Geometry check sheet. Reference: the model listing, model coordinates, mm. A direction names the side the tool comes from. Coordinates: 2 decimals unless noted, no trailing zeros. Loops run counter-clockwise (first coordinate to the right, second up) from the corner with the lowest first, then second, coordinate; pieces in that order, holes last. Notation, with made-up numbers: (28, 45) - (72, 45) arc R4 cw to (72, 50) - close; hole circle Ø6 at (24.25, 26). An arc over 180 degrees is marked (long way). Write item = value, one per line. Start each with the question number.
from build123d import *

# Parameters (mm, degrees)
SKETCH1_W                     = 114.3
SKETCH1_H                     = 254
BOSS_EXTRUDE1_DEPTH           = 2.000000064
M4_CLEARANCE_HOLE1_AT_2_COUNT = 2
M4_CLEARANCE_HOLE1_AT_2_PITCH = 64.13133097
M4_CLEARANCE_HOLE1_AT_3_COUNT = 2
M4_CLEARANCE_HOLE1_AT_3_PITCH = 171.44126128
M4_CLEARANCE_HOLE1_AT_4_COUNT = 2
M4_CLEARANCE_HOLE1_AT_4_PITCH = 158.994586252
SKETCH8_R                     = 6.35
BOSS_EXTRUDE3_DEPTH           = 3


with BuildPart() as part:
    # Sketch1 → Boss-Extrude1 (new body)
    with BuildSketch(Plane(origin=(0, 0, 0), x_dir=(1, 0, 0), z_dir=(0, 1, 0))):
        with Locations((57.15, 127)):
            Rectangle(SKETCH1_W, SKETCH1_H)
    extrude(amount=BOSS_EXTRUDE1_DEPTH)

    # Sketch6 → M4 Clearance Hole1 (revolve, cut)
    with BuildSketch(Plane(origin=(25.146, 2.000000064, -206.502), x_dir=(0, 0, 1), z_dir=(1, 0, 0))):
        Polygon((0, 0), (0, 2.000000064), (2.25, 2.000000064), (2.25, 0.025), (2.275, 0), align=None)
    m4_clearance_hole1 = revolve(axis=Axis((25.146, 8.350000064, -206.502), (0, -1, 0)), mode=Mode.SUBTRACT)

    # M4 Clearance Hole1 at 2: M4 Clearance Hole1 ×2
    with Locations(*[(i * M4_CLEARANCE_HOLE1_AT_2_PITCH, 0, 0) for i in range(1, M4_CLEARANCE_HOLE1_AT_2_COUNT)]):
        add(m4_clearance_hole1, mode=Mode.SUBTRACT)

    # M4 Clearance Hole1 at 3: M4 Clearance Hole1 ×2
    with Locations(*[Vector(0.37407174, 0, 0.92739977) * (i * M4_CLEARANCE_HOLE1_AT_3_PITCH) for i in range(1, M4_CLEARANCE_HOLE1_AT_3_COUNT)]):
        add(m4_clearance_hole1, mode=Mode.SUBTRACT)

    # M4 Clearance Hole1 at 4: M4 Clearance Hole1 ×2
    with Locations(*[(0, 0, i * M4_CLEARANCE_HOLE1_AT_4_PITCH) for i in range(1, M4_CLEARANCE_HOLE1_AT_4_COUNT)]):
        add(m4_clearance_hole1, mode=Mode.SUBTRACT)

    # Sketch8 → Boss-Extrude3 (add)
    with BuildSketch(Plane(origin=(0, 2.000000064, 0), x_dir=(1, 0, 0), z_dir=(0, 1, 0))):
        with Locations((89.27733097, 47.507413748)):
            Circle(SKETCH8_R)
        with BuildLine():
            ThreePointArc((89.228972354, 43.291716477), (89.012687116, 43.241374316), (88.800207525, 43.305919345))
            Line((88.800207525, 43.305919345), (85.540585246, 45.334637149))
            ThreePointArc((85.540585246, 45.334637149), (85.388845037, 45.496774579), (85.338502876, 45.713059817))
            Line((85.338502876, 45.713059817), (85.465612892, 49.55033442))
            ThreePointArc((85.465612892, 49.55033442), (85.53015792, 49.762814011), (85.692295351, 49.91455422))
            Line((85.692295351, 49.91455422), (89.079027646, 51.723111019))
            ThreePointArc((89.079027646, 51.723111019), (89.295312884, 51.77345318), (89.507792475, 51.708908151))
            Line((89.507792475, 51.708908151), (92.767414754, 49.680190347))
            ThreePointArc((92.767414754, 49.680190347), (92.919154963, 49.518052917), (92.969497124, 49.301767679))
            Line((92.969497124, 49.301767679), (92.842387108, 45.464493076))
            ThreePointArc((92.842387108, 45.464493076), (92.77784208, 45.252013485), (92.615704649, 45.100273276))
            Line((92.615704649, 45.100273276), (89.228972354, 43.291716477))
        make_face(mode=Mode.SUBTRACT)
        with Locations((25.02266903, 47.507413748)):
            Circle(SKETCH8_R)
        with BuildLine():
            Line((28.759414754, 45.334637149), (25.499792475, 43.305919345))
            ThreePointArc((25.499792475, 43.305919345), (25.287312884, 43.241374316), (25.071027646, 43.291716477))
            Line((25.071027646, 43.291716477), (21.684295351, 45.100273276))
            ThreePointArc((21.684295351, 45.100273276), (21.52215792, 45.252013485), (21.457612892, 45.464493076))
            Line((21.457612892, 45.464493076), (21.330502876, 49.301767679))
            ThreePointArc((21.330502876, 49.301767679), (21.380845037, 49.518052917), (21.532585246, 49.680190347))
            Line((21.532585246, 49.680190347), (24.792207525, 51.708908151))
            ThreePointArc((24.792207525, 51.708908151), (25.004687116, 51.77345318), (25.220972354, 51.723111019))
            Line((25.220972354, 51.723111019), (28.607704649, 49.91455422))
            ThreePointArc((28.607704649, 49.91455422), (28.76984208, 49.762814011), (28.834387108, 49.55033442))
            Line((28.834387108, 49.55033442), (28.961497124, 45.713059817))
            ThreePointArc((28.961497124, 45.713059817), (28.911154963, 45.496774579), (28.759414754, 45.334637149))
        make_face(mode=Mode.SUBTRACT)
        with Locations((89.27733097, 206.492586252)):
            Circle(SKETCH8_R)
        with BuildLine():
            Line((89.228972354, 210.708283523), (92.615704649, 208.899726724))
            ThreePointArc((92.615704649, 208.899726724), (92.77784208, 208.747986515), (92.842387108, 208.535506924))
            Line((92.842387108, 208.535506924), (92.969497124, 204.698232321))
            ThreePointArc((92.969497124, 204.698232321), (92.919154963, 204.481947083), (92.767414754, 204.319809653))
            Line((92.767414754, 204.319809653), (89.507792475, 202.291091849))
            ThreePointArc((89.507792475, 202.291091849), (89.295312884, 202.22654682), (89.079027646, 202.276888981))
            Line((89.079027646, 202.276888981), (85.692295351, 204.08544578))
            ThreePointArc((85.692295351, 204.08544578), (85.53015792, 204.237185989), (85.465612892, 204.44966558))
            Line((85.465612892, 204.44966558), (85.338502876, 208.286940183))
            ThreePointArc((85.338502876, 208.286940183), (85.388845037, 208.503225421), (85.540585246, 208.665362851))
            Line((85.540585246, 208.665362851), (88.800207525, 210.694080655))
            ThreePointArc((88.800207525, 210.694080655), (89.012687116, 210.758625684), (89.228972354, 210.708283523))
        make_face(mode=Mode.SUBTRACT)
        with Locations((25.02266903, 206.492586252)):
            Circle(SKETCH8_R)
        with BuildLine():
            ThreePointArc((25.071027646, 210.708283523), (25.287312884, 210.758625684), (25.499792475, 210.694080655))
            Line((25.499792475, 210.694080655), (28.759414754, 208.665362851))
            ThreePointArc((28.759414754, 208.665362851), (28.911154963, 208.503225421), (28.961497124, 208.286940183))
            Line((28.961497124, 208.286940183), (28.834387108, 204.44966558))
            ThreePointArc((28.834387108, 204.44966558), (28.76984208, 204.237185989), (28.607704649, 204.08544578))
            Line((28.607704649, 204.08544578), (25.220972354, 202.276888981))
            ThreePointArc((25.220972354, 202.276888981), (25.004687116, 202.22654682), (24.792207525, 202.291091849))
            Line((24.792207525, 202.291091849), (21.532585246, 204.319809653))
            ThreePointArc((21.532585246, 204.319809653), (21.380845037, 204.481947083), (21.330502876, 204.698232321))
            Line((21.330502876, 204.698232321), (21.457612892, 208.535506924))
            ThreePointArc((21.457612892, 208.535506924), (21.52215792, 208.747986515), (21.684295351, 208.899726724))
            Line((21.684295351, 208.899726724), (25.071027646, 210.708283523))
        make_face(mode=Mode.SUBTRACT)
    extrude(amount=BOSS_EXTRUDE3_DEPTH)


solid = part.part
(1) Sectioned sample at C-C on x = 64.5. Enter the section's corners in (y, z), plus the area to 3 significant figures.
(2) Scan lines: line 1 (Z direction, x = 89, y = 3.9); line 2 (Z direction, x = 92.5, y = 3.7); line 3 (Y direction, x = 79.5, z = -96). Record each from-to range of solid material in increasing order.
(3) Sectioned sample at B-B on y = 3.5. Count the separate pieces of the cut face and the enclosed holes in it, plus the area to 3 significant figures.
(4) Tool access check on faces 1 (the face through (27.34, 1, -48)), 2 (the face through (26.8, 2, -45.7)). Record the directions out of +Z, -Z, +X, -X, +Y, -Y that give a thin tool (end or side, any length) a straight path to the whole face; none if there is none.
(5) Sectioned sample at A-A on z = -226.5. Enter the section's corners in (x, y).
(6) Draft check along Z on faces 3 (the face through (18.68, 3.48, -47.79)), 4 (the face through (92, 5, -209.4)). Enter one of: pulls with the +Z half, pulls with the -Z half, needs draft (parallel to the pull), parting line crosses it, or undercut.
(7) Depth check by flat-ended pin: pin 1 (4 mm diameter, centred on x = 26.5, z = -206, fed in from +Y). Enter the tip coordinate at first touch or a pass-through.
Working result:
q1.outline = (0, -254) - (2, -254) - (2, 0) - (0, 0) - close
q1.area = 508 mm2
q2.line_1 = -212.84 to -210.76, -202.32 to -200.15, -53.85 to -51.68, -43.24 to -41.16
q2.line_2 = -211.96 to -208.96, -204.15 to -201.02, -52.98 to -49.85, -45.04 to -42.04
q2.line_3 = 0 to 2
q3.separate_pieces = 4
q3.enclosed_holes = 4
q3.area = 312 mm2
q4.face_1 = +Y, -Y
q4.face_2 = +Y
q5.outline = (0, 0) - (114.3, 0) - (114.3, 2) - (0, 2) - close
q6.face_3 = undercut
q6.face_4 = needs draft
q7.pin_1 = 2
